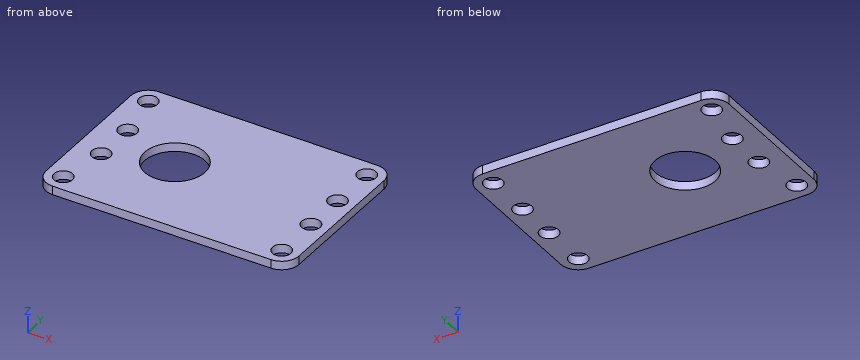
Autodesk Inventor part; units mm, degrees
ref_plane "YZ Plane" through (0, 0, 0) normal (1, 0, 0) x (0, 1, 0)
ref_plane "XZ Plane" through (0, 0, 0) normal (0, 1, 0) x (-1, 0, 0)
ref_plane "XY Plane" through (0, 0, 0) normal (0, 0, 1) x (1, 0, 0)
sketch "スケッチ1" plane through (0, 0, 0) normal (0, 0, 1) x (1, 0, 0)
  line L0 (-30, -20) -> (28.6, -20)
  line L1 (28.6, -20) -> (28.6, 20)
  line L2 (28.6, 20) -> (-30, 20)
  line L3 (-30, 20) -> (-30, -20)
  point P0 (0, 0)
  dimension "d1" = 40
  dimension "d28" = 30
  dimension "d29" = 28.6
  dimension "d32" = 20
extrude "プレート1" add sketch "スケッチ1" along normal blind 2
sketch "スケッチ2" plane through (0, 0, 2) normal (0, 0, 1) x (1, 0, 0)
  line L0 (-24, -5) -> (24.6, -5)
  line L1 (24.6, -5) -> (24.6, 5)
  line L2 (24.6, 5) -> (-24, 5)
  line L3 (-24, 5) -> (-24, -5)
  line L4 (-24, -5) -> (24.6, 5) construction
  line L5 (24.6, -5) -> (-24, 5) construction
  line L6 (28.6, -20) -> (-30, -20)
  line L7 (-30, -20) -> (-30, 20)
  line L8 (28.6, -20) -> (-30, -20)
  line L9 (28.6, 20) -> (28.6, -20)
  line L10 (-30, 20) -> (28.6, 20)
  circle A0 centre (-10, 0) radius 7
  point P0 (0.3, 0)
  point P1 (0.3, 0)
  point P2 (0.3, 0)
  point P3 (0, 0)
  dimension "d3" = 48.6
  dimension "d5" = 10
  dimension "d8" = 20
  dimension "d16" = 14
  dimension "d30" = 20
  dimension "d31" = 14
hole "穴1" at (24.6, 5, 2) at (24.6, -5, 2) at (-24, 5, 2) at (-24, -5, 2) direction (0, 0, -1) diameter 4.3 end through all
extrude "押し出し1" cut sketch "スケッチ2" against normal blind 10 contours A0 L2 L0 | L0 A0 | A0 L2
sketch "スケッチ3" plane through (0, 0, 2) normal (0, 0, 1) x (1, 0, 0)
  line L0 (-30, 20) -> (28.6, 20)
  line L1 (-30, -20) -> (-30, 20)
  line L2 (28.6, -20) -> (-30, -20)
  line L3 (28.6, 20) -> (28.6, -20)
  line L4 (24.6, 16) -> (-26, 16)
  line L5 (-26, 16) -> (-26, -16)
  line L6 (-26, -16) -> (24.6, -16)
  line L7 (24.6, -16) -> (24.6, 16)
  point P0 (0, 0)
  dimension "d19" = 4
hole "穴2" at (-26, 16, 2) at (-26, -16, 2) at (24.6, 16, 2) at (24.6, -16, 2) direction (0, 0, -1) diameter 4.3 end through all
fillet "コーナーR1" radius 4 4 edges at (28.6, 20, 1) (-30, 20, 1) (-30, -20, 1) (28.6, -20, 1)
equation "\"d14\" = Thickness"
equation "\"d2\" = Thickness"
equation "\"BendRadius\" = Thickness"
equation "\"BendReliefWidth\" = Thickness"
equation "\"BendReliefDepth\" = 0.5 * Thickness"
equation "\"CornerReliefSize\" = 4 * Thickness"
equation "\"MinimumRemnant\" = 2 * Thickness"
equation "\"TransitionRadius\" = BendRadius"
equation "\"JacobiRadiusSize\" = BendRadius"
equation "\"GapSize\" = Thickness"
properties part number "s_carbon_plate4" material "CFRP"
For this review, take the finished solid that the model builds, in its own axes (mm). Round coordinates to 2 decimals unless told otherwise and drop trailing zeros. Write each loop counter-clockwise with the first axis right and the second up, starting at its lowest first coordinate (ties: lowest second). Pieces come first, ordered by that corner, then holes. Notation, with made-up numbers: (76.5, 67) -> (134.5, 67) arc R11 ccw to (134.5, 81) -> close; hole circle Ø5 at (3, 31). An arc over 180 degrees is marked (long way). One line per question, with ' | ' between items. Start each with the question number.
(1) Insertion check: P1, Ø4, axis at x = -26, y = 16, coming from the -Z side. The pin has a flat end and moves straight along its axis. Give the tip position at first contact, or say it passes through.
(2) Add section B-B, the plane y = 2. Write out the cut boundary in (x, z), plus the area to 3 significant figures.
(3) Add section C-C, the plane y = -5. Write out the cut boundary in (x, z), plus the area to 3 significant figures.
(4) For line 1 along Y through (x, z) = (24.6, 0.4); line 2 along X through (y, z) = (-17, 0.8); line 3 along X through (y, z) = (-3.5, 1.55), list the stretches that pass through material, from the lowest coordinate up. Write a range as from..to.
(5) Add section A-A, the plane z = 0.95. Give the number of separate pieces and of enclosed holes in the cut face, plus the area to 3 significant figures.
(6) Add section D-D, the plane y = 14.5. Write out the cut boundary in (x, z).
Answer list:
1) P1: through
2) outline: (-30, 0) -> (-16.71, 0) -> (-16.71, 2) -> (-30, 2) -> close; (-3.29, 0) -> (28.6, 0) -> (28.6, 2) -> (-3.29, 2) -> close | area: 90.4 mm²
3) outline: (-30, 0) -> (-26.15, 0) -> (-26.15, 2) -> (-30, 2) -> close; (-21.85, 0) -> (-14.9, 0) -> (-14.9, 2) -> (-21.85, 2) -> close; (-5.1, 0) -> (22.45, 0) -> (22.45, 2) -> (-5.1, 2) -> close; (26.75, 0) -> (28.6, 0) -> (28.6, 2) -> (26.75, 2) -> close | area: 80.4 mm²
4) line 1: -20..-18.15, -13.85..-7.15, -2.85..2.85, 7.15..13.85, 18.15..20 | line 2: -29.87..-27.9, -24.1..22.7, 26.5..28.47 | line 3: -30..-25.54, -22.46..-16.06, -3.94..23.06, 26.14..28.6
5) separate pieces: 1 | enclosed holes: 9 | area: 2,060 mm²
6) outline: (-30, 0) -> (-27.54, 0) -> (-27.54, 2) -> (-30, 2) -> close; (-24.46, 0) -> (23.06, 0) -> (23.06, 2) -> (-24.46, 2) -> close; (26.14, 0) -> (28.6, 0) -> (28.6, 2) -> (26.14, 2) -> close
